from build123d import *

# Parameters (mm, degrees)
BALAYAGE_MINCE1_PROFILE_R   = 3
BALAYAGE_MINCE1_PROFILE_R_2 = 2


with BuildPart() as part:
    # Balayage-Mince1: sweep along a curve in space
    with BuildLine() as balayage_mince1_path:
        Line((-42, 165, -59.25), (-42, 195.275, -59.25))
        ThreePointArc((-42, 195.275, -59.25), (-3, 234.443107243, -55.625), (36, 195.275, -52))
        Line((36, 195.275, -52), (36, 109.55, -52))
    # Balayage-Mince1 profile (on start of the path) → Balayage-Mince1 (sweep)
    with BuildSketch(Plane(origin=(-42, 165, -59.25), x_dir=(0, 0, 1), z_dir=(0, 1, 0))):
        Circle(BALAYAGE_MINCE1_PROFILE_R)
        Circle(BALAYAGE_MINCE1_PROFILE_R_2, mode=Mode.SUBTRACT)
    sweep(path=balayage_mince1_path.line)


solid = part.part
The listing builds one solid part. Answer for the finished solid, in the listing's coordinates (mm). A direction names the side the tool comes from. Round coordinates to 2 decimals unless told otherwise and drop trailing zeros. Write each loop counter-clockwise with the first axis right and the second up, starting at its lowest first coordinate (ties: lowest second). Pieces come first, ordered by that corner, then holes. Notation, with made-up numbers: M 26,16.5 L 57,16.5 A21 ccw 57,37.5 Z; hole C 8.5,-36.5 d1. An arc over 180 degrees is marked long. Write each question's results on one line, items separated by ' | '. Start each with the question number.
Item 1: The mould has two halves that part along X. Classify faces 1 (the flat face through (-43, 165, -57)), 2 (the cylindrical face through (34.59, 151.81, -49.35)), 3 (the cylindrical face through (-43.774, 180.349, -58.327)), 4 (the cylindrical face through (34.943, 151.812, -53.698)): +X half, -X half, draft (parallel to the pull), parting line (faces both ways), or undercut.
Item 2: Given pin 1 Ø3 at (y, z) = (185.5, -54.5) entering from +X; pin 2 Ø1.5 at (y, z) = (189.5, -60.5) entering from -X; pin 3 Ø3 at (x, z) = (-41.5, -58) entering from -Y, each flat-ended and moving along its own axis, determine where each tip first touches the part or whether it passes through.
Item 3: Find section C-C on y = 215. Give the number of separate pieces and of enclosed holes in the cut face, and give its area (3 significant figures).
Item 4: Find section A-A on y = 174. Write down the section's boundary in (x, z).
Item 5: Which of the six approach directions +Z, -Z, +X, -X, +Y, -Y give full straight-line access (tool end or side, diameter ignored) to faces 5 (the flat face through (35, 109.55, -54)), 6 (the cylindrical face through (-39.97, 180.35, -61.46))?
Item 6: Straight lines are drawn through the part: probe 1 along X at (y, z) = (156, -52); probe 2 along Z at (x, y) = (36, 165.5); probe 3 along X at (y, z) = (186, -59.25). For each, find the intervals that lie inside material, in ascending order.
Item 7: Find section B-B on y = 145.5. Write down the section's boundary in (x, z), and give its area (3 significant figures).
Answer block:
1) face 1: draft | face 2: parting line | face 3: undercut | face 4: undercut
2) pin 1: stops at x = 38.83 | pin 2: stops at x = -44.96 | pin 3: stops at y = 165
3) separate pieces: 2 | enclosed holes: 2 | area: 36.4 mm²
4) outline: C -42,-59.25 d6; C 36,-52 d6; hole C -42,-59.25 d4; hole C 36,-52 d4
5) face 5: +Z, -Z, +X, -X, -Y | face 6: -Y
6) probe 1: x = 33 to 34, 38 to 39 | probe 2: z = -55 to -54, -50 to -49 | probe 3: x = -45 to -44, -40 to -39
7) outline: C 36,-52 d6; hole C 36,-52 d4 | area: 15.7 mm²
